Model file for the job. Use its own axes, mm. Round coordinates to 2 decimals unless told otherwise and drop trailing zeros. Order: outer loops, then holes, each group sorted by start corner. A loop starts at its lowest first (then second) coordinate and runs counter-clockwise, first axis right, second up. Notation, with made-up numbers: (84, 14) -> (117, 14) arc R26 ccw to (117, 42) -> close; hole circle Ø1 at (-28, 16). An arc over 180 degrees is marked (long way). Use CSV: the item, a comma, the result in double quotes.
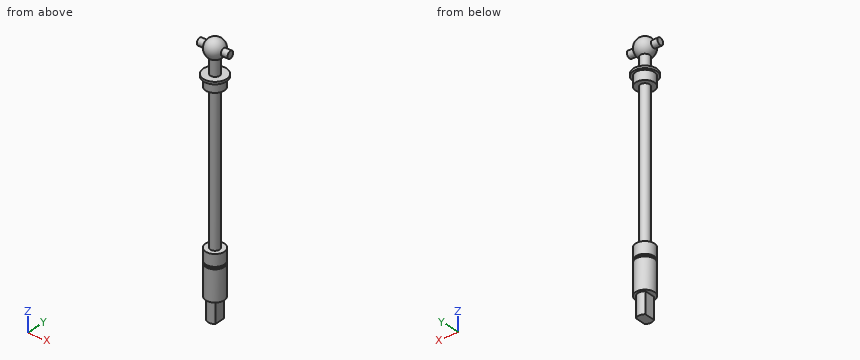
```python
from build123d import *

# Parameters (mm, degrees)
CUT_EXTRUDE1_DEPTH  = 9
SKETCH3_R           = 1.5
BOSS_EXTRUDE1_DEPTH = 6.5


with BuildPart() as part:
    # Sketch1 → Revolve1 (revolve)
    with BuildSketch(Plane(origin=(0, 0, 0), x_dir=(0, 0, -1), z_dir=(1, 0, 0))):
        with BuildLine():
            Line((7.464101615, 2), (14, 2))
            Line((14, 2), (14, 5))
            Line((14, 5), (15, 5))
            Line((15, 5), (15, 4))
            Line((15, 4), (19, 4))
            Line((19, 4), (19, 2))
            Line((19, 2), (82, 2))
            Line((82, 2), (82, 4))
            Line((82, 4), (87, 4))
            Line((87, 4), (87, 3.5))
            Line((87, 3.5), (88, 3.5))
            Line((88, 3.5), (88, 4))
            Line((88, 4), (101, 4))
            Line((101, 4), (101, 3))
            Line((101, 3), (110, 3))
            Line((110, 3), (110, 0))
            Line((110, 0), (0, 0))
            ThreePointArc((0, 0), (2.96472382, 3.863703305), (7.464101615, 2))
        make_face()
    revolve(axis=Axis((0, 0, 0), (0, 0, -1)))

    # Sketch2 → Cut-Extrude1 (cut)
    with BuildSketch(Plane(origin=(0, 0, -110), x_dir=(-1, 0, 0), z_dir=(0, 0, -1))):
        with BuildLine():
            ThreePointArc((-2, 2.236067977), (-3, 0), (-2, -2.236067977))
            Line((-2, -2.236067977), (-2, 2.236067977))
        make_face()
        with BuildLine():
            Line((2, 2.236067977), (2, -2.236067977))
            ThreePointArc((2, -2.236067977), (2.738612788, -1.224744871), (3, 0))
            ThreePointArc((3, 0), (2.738612788, 1.224744871), (2, 2.236067977))
        make_face()
    extrude(amount=-CUT_EXTRUDE1_DEPTH, mode=Mode.SUBTRACT)

    # Sketch3 → Boss-Extrude1 (add, symmetric)
    with BuildSketch(Plane(origin=(0, 0, 0), x_dir=(0, 0, -1), z_dir=(1, 0, 0))):
        with Locations((4, 0)):
            Circle(SKETCH3_R)
    extrude(amount=BOSS_EXTRUDE1_DEPTH, both=True)


solid = part.part
```
Q1. Cut at A-A (z = -4). Give the cut face in (x, y).
From the geometry:
outline,"(-6.5, -1.5) -> (-3.71, -1.5) arc R4 ccw to (3.71, -1.5) -> (6.5, -1.5) -> (6.5, 1.5) -> (3.71, 1.5) arc R4 ccw to (-3.71, 1.5) -> (-6.5, 1.5) -> close"
Q2. Cut at C-C (z = -18). Give the cut face in (x, y), plus the area to 3 significant figures.
From the geometry:
outline,"circle Ø8 at (0, 0)"
area,"50.3 mm²"
Q3. Cut at B-B (z = -33). Give the cut face in (x, y), plus the area to 3 significant figures.
From the geometry:
outline,"circle Ø4 at (0, 0)"
area,"12.6 mm²"
Q4. Probe line 1 along Z through (x, y) = (3, -2); line 2 along Z through (x, y) = (1.5, -1.75); line 3 along Z through (x, y) = (-2.75, -0.25). List the from-to ranges inside material, lowest first.
From the geometry:
line 1,"z = -101 to -88, -87 to -82, -19 to -14, -5.73 to -2.27"
line 2,"z = -110 to -82, -19 to -14, -7.27 to -0.73"
line 3,"z = -101 to -82, -19 to -14, -6.89 to -1.11"
Q5. Pin check, flat tips, straight feed: pin 1 (2 mm diameter, centred on y = 1.5, z = -88, fed in from +X); pin 2 (1.5 mm diameter, centred on x = 1, z = -21.5, fed in from -Y); pin 3 (5 mm diameter, centred on x = 0.5, y = 0, fed in from +Z); pin 4 (5 mm diameter, centred on y = -1, z = -107, fed in from -X). Stop position of each tip, or through.
From the geometry:
pin 1,"stops at x = 3.97"
pin 2,"stops at y = -1.98"
pin 3,"stops at z = 0"
pin 4,"stops at x = -2"
